Build history of the part. All positions in model axes, mm. A direction names the side the tool comes from. Round coordinates to 2 decimals unless told otherwise and drop trailing zeros. Write each loop counter-clockwise with the first axis right and the second up, starting at its lowest first coordinate (ties: lowest second). Pieces come first, ordered by that corner, then holes. Notation, with made-up numbers: (-34, -38) - (-23, -38) arc R30 cw to (-23, -6) - close; hole circle Ø7 at (65.25, 62.5). An arc over 180 degrees is marked (long way). Answer as a JSON object with one key per item and string values. Group by question number.
Item 1: Probe line 1 (Y direction, x = -41.25, z = 0.65); line 2 (X direction, y = 33, z = 0.7); line 3 (Y direction, x = 44.15, z = -0.25). List the from-to ranges inside material, lowest first. Write a range as from..to.
Item 2: Which spindle directions (+Z, -Z, +X, -X, +Y, -Y) get a long thin tool onto all of the face, cutting with end or side? Do faces 5 (the flat face through (-49.5, 44, 0)), 6 (the cylindrical face through (-51, 49, 0)). Say none if no direction does.
Item 3: Slice it at B-B, the plane y = -10.5. List the corners of the cut face in (x, z).
Item 4: Flat gauge pins, fed straight in: pin 1 (0.9 mm diameter, centred on y = 12, z = -0.5, fed in from +X); pin 2 (1.5 mm diameter, centred on x = 13.5, z = 0, fed in from -Y); pin 3 (0.9 mm diameter, centred on y = -3.5, z = 0.5, fed in from -X). Where does each tip first touch, or does it go through?
Item 5: Slice it at D-D, the plane z = -0.2. Give the number of separate pieces and of enclosed holes in the cut face, then the cut area to 3 significant figures.
Item 6: Two-plate mould, pull along X, no slides. Class faces 1 (the flat face through (10.5, -7, 0)), 2 (the cylindrical face through (52, 48, 0)), 3 (the flat face through (20, -49, 0)), 4 (the flat face through (-1, 1, 1.5)): +X half, -X half, draft (parallel to the pull), parting line (faces both ways), or undercut.
Item 7: Slice it at A-A, the plane x = 27. List the corners of the cut face in (y, z), then the cut area to 3 significant figures.
Item 8: Slice it at C-C, the plane y = 11.5. List the corners of the cut face in (x, z), then the cut area to 3 significant figures.
from build123d import *

# Parameters (mm, degrees)
ESBO_O1_W                 = 100
ESBO_O1_H                 = 100
RESSALTO_EXTRUS_O1_DEPTH  = 1.5
ESBO_O2_R                 = 1.5
ESBO_O2_W                 = 40
ESBO_O2_H                 = 3
CORTE_EXTRUS_O1_DEPTH     = 4
ESBO_O3_W                 = 3
ESBO_O3_H                 = 34.5
RESSALTO_EXTRUS_O2_DEPTH  = 3
CUT_EXTRUDE4_DEPTH        = 2.5
CUT_EXTRUDE4_DEPTH_BACK   = 2.5
FILLET1_R                 = 5
SKETCH3_W                 = 3
SKETCH3_H                 = 15
SKETCH3_W_2               = 4
SKETCH3_H_2               = 3
CUT_EXTRUDE5_DEPTH        = 2.5
CUT_EXTRUDE5_DEPTH_BACK   = 2.5
SKETCH8_R                 = 1.5
SKETCH8_W                 = 11.5
SKETCH8_H                 = 3
CORTE_GY_53LDK_DEPTH      = 2.5
CORTE_GY_53LDK_DEPTH_BACK = 2.5
SKETCH4_R                 = 1.1
SKETCH4_W                 = 22.5
SKETCH4_H                 = 12.2
CUT_EXTRUDE6_DEPTH        = 1
CUT_EXTRUDE6_DEPTH_BACK   = 4
CUT_EXTRUDE7_DEPTH        = 1
CUT_EXTRUDE7_DEPTH_BACK   = 4


with BuildPart() as part:
    # Esboço1 → Ressalto-extrusão1 (new body, symmetric)
    with BuildSketch(Plane.XY):
        Rectangle(ESBO_O1_W, ESBO_O1_H)
    extrude(amount=RESSALTO_EXTRUS_O1_DEPTH, both=True)

    # Esboço2 → Corte-extrusão1 (cut, through all)
    with BuildSketch(Plane.XY.offset(1.5)):
        with Locations((-33, 11.5)):
            Circle(ESBO_O2_R)
        with Locations((33, 11.5)):
            Circle(ESBO_O2_R)
        with Locations((0, -48.5)):
            Rectangle(ESBO_O2_W, ESBO_O2_H)
        with Locations((0, 11.5)):
            Rectangle(ESBO_O2_W, ESBO_O2_H)
    extrude(amount=-CORTE_EXTRUS_O1_DEPTH, mode=Mode.SUBTRACT)

    # Esboço3 → Ressalto-extrusão2 (add, through all)
    with BuildSketch(Plane.XY.offset(1.5)):
        with Locations((-51.5, -32.75)):
            Rectangle(ESBO_O3_W, ESBO_O3_H)
        with Locations((51.5, -32.75)):
            Rectangle(ESBO_O3_W, ESBO_O3_H)
        with Locations((-51.5, 32.75)):
            Rectangle(ESBO_O3_W, ESBO_O3_H)
        with Locations((51.5, 32.75)):
            Rectangle(ESBO_O3_W, ESBO_O3_H)
    extrude(amount=-RESSALTO_EXTRUS_O2_DEPTH)

    # Sketch2 → Cut-Extrude4 (cut, two sides)
    with BuildSketch(Plane.XY) as cut_extrude4_sk:
        with BuildLine():
            Line((-0.5, -35), (0.5, -35))
            ThreePointArc((0.5, -35), (1.207106781, -35.292893219), (1.5, -36))
            Line((1.5, -36), (1.5, -40.73))
            Line((1.5, -40.73), (2.85, -40.73))
            Line((2.85, -40.73), (2.85, -43))
            Line((2.85, -43), (1.5, -43))
            Line((1.5, -43), (1.5, -47))
            Line((1.5, -47), (-1.5, -47))
            Line((-1.5, -47), (-1.5, -43))
            Line((-1.5, -43), (-2.85, -43))
            Line((-2.85, -43), (-2.85, -40.73))
            Line((-2.85, -40.73), (-1.5, -40.73))
            Line((-1.5, -40.73), (-1.5, -36))
            ThreePointArc((-1.5, -36), (-1.207106781, -35.292893219), (-0.5, -35))
        make_face()
    extrude(amount=CUT_EXTRUDE4_DEPTH, mode=Mode.SUBTRACT)
    extrude(cut_extrude4_sk.sketch, amount=-CUT_EXTRUDE4_DEPTH_BACK, mode=Mode.SUBTRACT)

    # Fillet1
    fillet1_edges = [part.edges().sort_by_distance(p)[0] for p in [
        (53, 50, 0),
        (-53, 50, 0),
    ]]
    fillet(fillet1_edges, radius=FILLET1_R)

    # Sketch3 → Cut-Extrude5 (cut, two sides)
    with BuildSketch(Plane.XY) as cut_extrude5_sk:
        with Locations((9, -6.5)):
            Rectangle(SKETCH3_W, SKETCH3_H)
        with Locations((9, 28.5)):
            Rectangle(SKETCH3_W, SKETCH3_H)
        with Locations((-9, 28.5)):
            Rectangle(SKETCH3_W, SKETCH3_H)
        with Locations((-9, -6.5)):
            Rectangle(SKETCH3_W, SKETCH3_H)
        with Locations((0, -27.5)):
            Rectangle(SKETCH3_W_2, SKETCH3_H_2)
        Polygon((-15.196152423, -40), (-10, -37), (-8.5, -39.598076211), (-13.696152423, -42.598076211), align=None)
        Polygon((10, -37), (8.5, -39.598076211), (13.696152423, -42.598076211), (15.196152423, -40), align=None)
    extrude(amount=CUT_EXTRUDE5_DEPTH, mode=Mode.SUBTRACT)
    extrude(cut_extrude5_sk.sketch, amount=-CUT_EXTRUDE5_DEPTH_BACK, mode=Mode.SUBTRACT)

    # Sketch8 → Corte GY-53LDK (cut, two sides)
    with BuildSketch(Plane.XY) as corte_gy_53ldk_sk:
        with Locations((-41.25, 35.2)):
            Circle(SKETCH8_R)
        with Locations((46.25, 35.2)):
            Circle(SKETCH8_R)
        with Locations((-43.75, 44.5)):
            Rectangle(SKETCH8_W, SKETCH8_H)
        with Locations((43.75, 44.5)):
            Rectangle(SKETCH8_W, SKETCH8_H)
    extrude(amount=CORTE_GY_53LDK_DEPTH, mode=Mode.SUBTRACT)
    extrude(corte_gy_53ldk_sk.sketch, amount=-CORTE_GY_53LDK_DEPTH_BACK, mode=Mode.SUBTRACT)

    # Sketch4 → Cut-Extrude6 (cut, two sides)
    with BuildSketch(Plane.XY.offset(1.5)) as cut_extrude6_sk:
        with Locations((44.15, -2.75)):
            Circle(SKETCH4_R)
        with Locations((16.35, -2.75)):
            Circle(SKETCH4_R)
        with Locations((30.25, -2.75)):
            Rectangle(SKETCH4_W, SKETCH4_H)
    extrude(amount=CUT_EXTRUDE6_DEPTH, mode=Mode.SUBTRACT)
    extrude(cut_extrude6_sk.sketch, amount=-CUT_EXTRUDE6_DEPTH_BACK, mode=Mode.SUBTRACT)

    # Sketch6 → Cut-Extrude7 (cut, two sides)
    with BuildSketch(Plane.XY.offset(1.5)) as cut_extrude7_sk:
        with BuildLine():
            Line((-31.2, -20.5), (-6.2, -20.5))
            ThreePointArc((-6.2, -20.5), (-4.7, -22), (-6.2, -23.5))
            Line((-6.2, -23.5), (-31.2, -23.5))
            ThreePointArc((-31.2, -23.5), (-32.7, -22), (-31.2, -20.5))
        make_face()
        with BuildLine():
            Line((6.2, -17), (31.2, -17))
            ThreePointArc((31.2, -17), (32.7, -18.5), (31.2, -20))
            Line((31.2, -20), (6.2, -20))
            ThreePointArc((6.2, -20), (4.7, -18.5), (6.2, -17))
        make_face()
    extrude(amount=CUT_EXTRUDE7_DEPTH, mode=Mode.SUBTRACT)
    extrude(cut_extrude7_sk.sketch, amount=-CUT_EXTRUDE7_DEPTH_BACK, mode=Mode.SUBTRACT)


solid = part.part
Geometry says:
{
 "1": {"line 1": "y = -50..33.7, 36.7..43, 46..50", "line 2": "x = -53..-10.5, -7.5..7.5, 10.5..53", "line 3": "y = -50..-3.85, -1.65..43, 46..50"},
 "2": {"face 5": "+Z, -Z", "face 6": "+Z, -Z, -X, +Y"},
 "3": {"outline": "(-50, -1.5) - (-10.5, -1.5) - (-10.5, 1.5) - (-50, 1.5) - close; (-7.5, -1.5) - (7.5, -1.5) - (7.5, 1.5) - (-7.5, 1.5) - close; (10.5, -1.5) - (50, -1.5) - (50, 1.5) - (10.5, 1.5) - close"},
 "4": {"pin 1": "stops at x = 50", "pin 2": "stops at y = -47", "pin 3": "stops at x = -50"},
 "5": {"separate pieces": "1", "enclosed holes": "19", "area": "9,350 mm^2"},
 "6": {"face 1": "undercut", "face 2": "+X half", "face 3": "undercut", "face 4": "draft"},
 "7": {"outline": "(-50, -1.5) - (-20, -1.5) - (-20, 1.5) - (-50, 1.5) - close; (-17, -1.5) - (-8.85, -1.5) - (-8.85, 1.5) - (-17, 1.5) - close; (3.35, -1.5) - (50, -1.5) - (50, 1.5) - (3.35, 1.5) - close", "area": "254 mm^2"},
 "8": {"outline": "(-50, -1.5) - (-34.5, -1.5) - (-34.5, 1.5) - (-50, 1.5) - close; (-31.5, -1.5) - (-20, -1.5) - (-20, 1.5) - (-31.5, 1.5) - close; (20, -1.5) - (31.5, -1.5) - (31.5, 1.5) - (20, 1.5) - close; (34.5, -1.5) - (50, -1.5) - (50, 1.5) - (34.5, 1.5) - close", "area": "162 mm^2"}
}
